from build123d import *

# Parameters (mm, degrees)
SCHIZZO1_R             = 26
ESTRUSIONE1_DEPTH      = 50
SCHIZZO2_R             = 10
ESTRUSIONE2_DEPTH      = 86
SMUSSO1_SIZE           = 2
ESTRUSIONE3_DEPTH      = 141.882930123
ESTRUSIONE3_DEPTH_BACK = 141.882930123
SCHIZZO3_R             = 4
SMUSSO2_SIZE           = 2


with BuildPart() as part:
    # Schizzo1 → Estrusione1 (new body)
    with BuildSketch(Plane.XY):
        Circle(SCHIZZO1_R)
    extrude(amount=ESTRUSIONE1_DEPTH)

    # Schizzo2 → Estrusione2 (add)
    with BuildSketch(Plane.XY.offset(50)):
        Circle(SCHIZZO2_R)
    extrude(amount=ESTRUSIONE2_DEPTH)

    # Smusso1
    smusso1_edges = [part.edges().sort_by_distance(p)[0] for p in [
        (-10, 0, 136),
    ]]
    chamfer(smusso1_edges, length=SMUSSO1_SIZE)

    # Schizzo3 → Estrusione3 (cut, two sides: drawn at the far end of the back side and taken through both)
    with BuildSketch(Plane(origin=(0, 0, 0), x_dir=(1, 0, 0), z_dir=(0, 1, 0)).offset(-ESTRUSIONE3_DEPTH_BACK)):
        with Locations(Location((0, -126, 0), (0, 0, 270))):
            Circle(SCHIZZO3_R)
    extrude(amount=ESTRUSIONE3_DEPTH + ESTRUSIONE3_DEPTH_BACK, mode=Mode.SUBTRACT)

    # Smusso2
    smusso2_edges = [part.edges().sort_by_distance(p)[0] for p in [
        (-26, 0, 0),
    ]]
    chamfer(smusso2_edges, length=SMUSSO2_SIZE)


solid = part.part
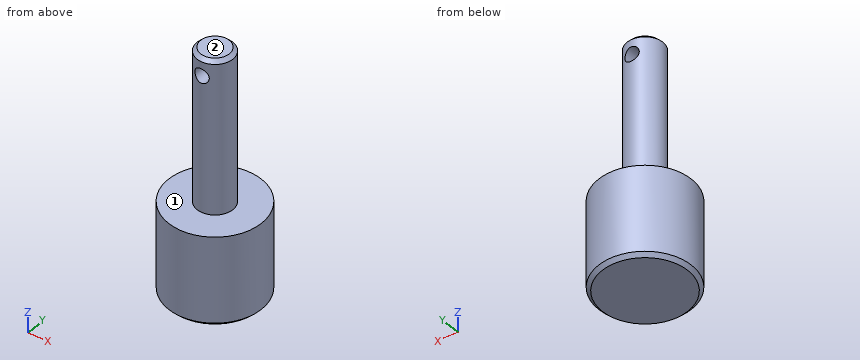
Geometry check sheet. Reference: the model listing, model coordinates, mm. Face numbers are marked on the shaded views. A direction names the side the tool comes from. Give positions to 0.01 mm unless a question says otherwise; leave off trailing zeros. Write each loop counter-clockwise with the first axis right and the second up, starting at its lowest first coordinate (ties: lowest second). Pieces come first, ordered by that corner, then holes. Notation, with made-up numbers: M 35,12.25 L 77,12.25 A13 ccw 77,32.25 Z; hole C 17.25,7.5 d9. An arc over 180 degrees is marked long. Answer as CSV lines item,"result". Start each with the question number.
Q1. Go/stop test with flat-tipped pins: pin 1 (1 mm diameter, centred on x = 12, z = 86, fed in from -Y); pin 2 (8 mm diameter, centred on x = -14, y = 10, fed in from +Z); pin 3 (10.5 mm diameter, centred on x = 0, z = 126, fed in from +Y); pin 4 (8 mm diameter, centred on x = -13, z = 72, fed in from -Y). Record where each tip stops, or that it passes through.
Q2. Section check C-C, the plane z = 22.5. Record the cut outline in (x, y).
Q3. Section check A-A, the plane x = 0. Record the cut outline in (y, z).
Q4. Tool access check on the marked faces 1 and 2. Record the directions out of +Z, -Z, +X, -X, +Y, -Y that give a thin tool (end or side, any length) a straight path to the whole face; none if there is none.
Q5. Section check D-D, the plane z = 126. Record the cut outline in (x, y).
Q6. Material ranges on L1, parallel to Z at x = 0, y = -5; L2, parallel to X at y = 3, z = 126; L3, parallel to Z at x = -16, y = -2.5, recorded low to high.
Q7. Section check B-B, the plane y = 0. Record the cut outline in (x, z).
Geometry says:
1,pin 1,"through"
1,pin 2,"z = 50"
1,pin 3,"y = 10"
1,pin 4,"y = -4.36"
2,outline,"C 0,0 d52"
3,outline,"M -26,2 L -24,0 L 24,0 L 26,2 L 26,50 L 10,50 L 10,122 L -10,122 L -10,50 L -26,50 Z; M -10,130 L 10,130 L 10,134 L 8,136 L -8,136 L -10,134 Z"
4,face 1,"+Z"
4,face 2,"+Z, +X, -X, +Y, -Y"
5,outline,"M -4,-9.17 L -4,9.17 A10 ccw Z; M 4,-9.17 A10 ccw 4,9.17 Z"
6,L1,"0 to 122, 130 to 136"
6,L2,"-9.54 to -4, 4 to 9.54"
6,L3,"0 to 50"
7,outline,"M -26,2 L -24,0 L 24,0 L 26,2 L 26,50 L 10,50 L 10,134 L 8,136 L -8,136 L -10,134 L -10,50 L -26,50 Z; hole C 0,126 d8"
